Verification items for this drawing (mm, ordinates from the low corner). A direction names the side the tool comes from. Round coordinates to 2 decimals unless told otherwise and drop trailing zeros. Write each loop counter-clockwise with the first axis right and the second up, starting at its lowest first coordinate (ties: lowest second). Pieces come first, ordered by that corner, then holes.
Item 1: Access from +Z, -Z, +X, -X, +Y, -Y to the whole of each face (thin tool, end or side, straight path). Record for the marked faces 1 and 2.
Item 2: Cross-section at A-A (x = 10). Enter the section's corners in (y, z).
Item 3: Cross-section at C-C (z = 8). Enter the section's corners in (x, y).
Item 4: Scan lines: probe 1 along Z at (x, y) = (9.5, 2); probe 2 along Z at (x, y) = (7, 11.25); probe 3 along Y at (x, z) = (16.5, 0.5). Record each from-to range of solid material in increasing order.
Item 5: Depth check by flat-ended pin: P1, Ø5, axis at x = 13, z = 10, coming from the -Y side (3 decimals); P2, Ø5, axis at y = 16.5, z = 2.5, coming from the +X side; P3, Ø6, axis at y = 2.5, z = 2, coming from the -X side. Enter the tip coordinate at first touch or a pass-through.
Item 6: Cross-section at D-D (z = 1.25). Enter the section's corners in (x, y), then the cut area to 3 significant figures.
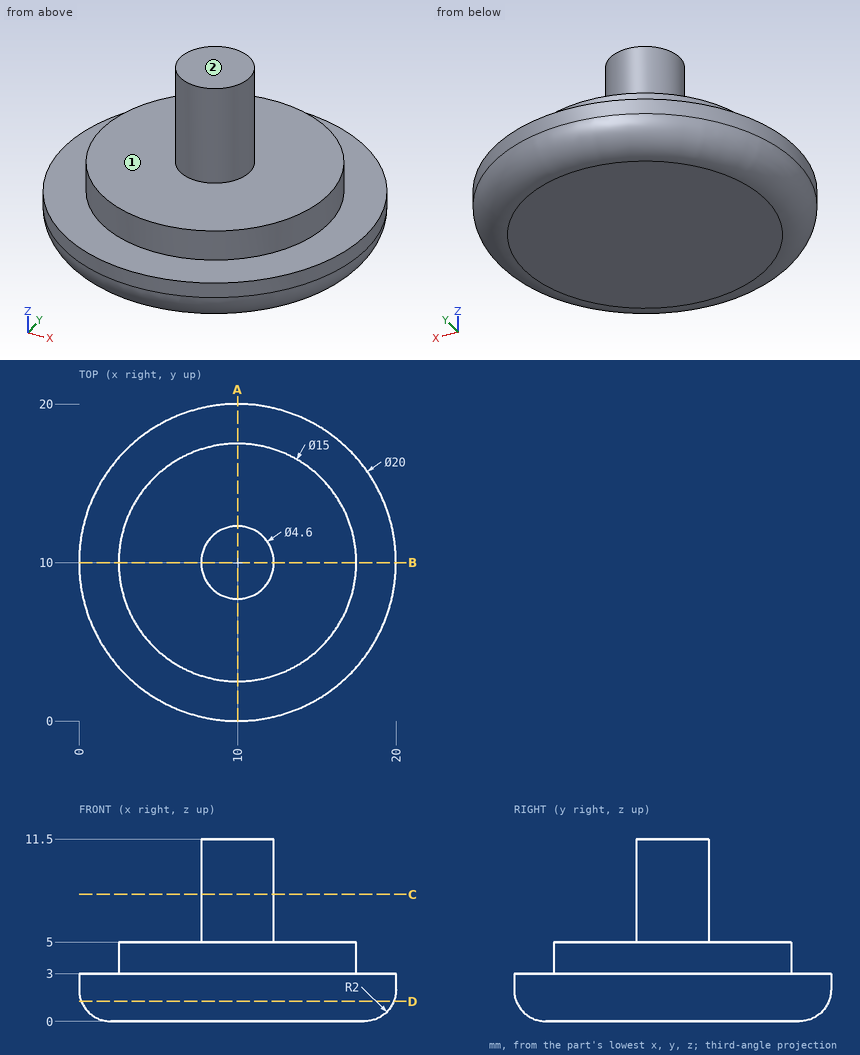
Resolved:
1. face 1: +Z
1. face 2: +Z, +X, -X, +Y, -Y
2. outline: (0, 2) arc R2 ccw to (2, 0) - (18, 0) arc R2 ccw to (20, 2) - (20, 3) - (17.5, 3) - (17.5, 5) - (12.3, 5) - (12.3, 11.5) - (7.7, 11.5) - (7.7, 5) - (2.5, 5) - (2.5, 3) - (0, 3) - close
3. outline: circle Ø4.6 at (10, 10)
4. probe 1: z = 0 to 3
4. probe 2: z = 0 to 5
4. probe 3: y = 3.32 to 16.68
5. P1: stops at y = 7.755
5. P2: stops at x = 19.17
5. P3: stops at x = 1.07
6. outline: circle Ø19.71 at (10, 10)
6. area: 305 mm2
